```python
from build123d import *

# Parameters (mm, degrees)
SKETCH_W     = 13
SKETCH_H     = 10
PAD_DEPTH    = 12
POCKET_DEPTH = 8.5
SKETCH002_W  = 3
SKETCH002_H  = 10
PAD001_DEPTH = 10


with BuildPart() as part:
    # Sketch → Pad (new body)
    with BuildSketch(Plane.XZ):
        with Locations((0, -3)):
            Rectangle(SKETCH_W, SKETCH_H)
    extrude(amount=PAD_DEPTH)

    # Sketch001 → Pocket (cut)
    with BuildSketch(Plane(origin=(0, 0, 0), x_dir=(-1, 0, 0), z_dir=(0, 1, 0))):
        Polygon((-1.5, 5.906373), (1.5, 5.906373), (1.5, 0), (4.65, 0), (4.65, -8.83584), (-4.65, -8.83584), (-4.65, 0), (-1.5, 0), align=None)
    extrude(amount=-POCKET_DEPTH, mode=Mode.SUBTRACT)

    # Sketch002 (on Face7 of Pocket) → Pad001 (join)
    with BuildSketch(Plane(origin=(6.5, 0, 0), x_dir=(0, 0, 1), z_dir=(1, 0, 0))):
        with Locations((-6.5, 6)):
            Rectangle(SKETCH002_W, SKETCH002_H)
    pad001 = extrude(amount=PAD001_DEPTH)

    # Sketch003 (on DatumPlane) → Groove (revolve, cut)
    with BuildSketch(Plane.YZ.offset(11.5)):
        Polygon((-6, -5), (-8.636665, -5), (-7.5, -6.55), (-7.5, -10.559105), (-6, -10.559105), align=None)
    groove = revolve(axis=Axis((11.5, -6, -3.810725), (0, 0, -1)), mode=Mode.SUBTRACT)

    # Mirrored: Pad001, Groove across YZ
    add(pad001.mirror(Plane.YZ))
    add(groove.mirror(Plane.YZ), mode=Mode.SUBTRACT)


solid = part.part
```
Geometry check sheet. Reference: the model listing, model coordinates, mm. A direction names the side the tool comes from. Give positions to 0.01 mm unless a question says otherwise; leave off trailing zeros. Order: outer loops, then holes, each group sorted by start corner. A loop starts at its lowest first (then second) coordinate and runs counter-clockwise, first axis right, second up. Notation, with made-up numbers: (-29.5, 53) - (-11.5, 53) arc R22 cw to (-11.5, 89) - close; hole circle Ø3 at (-38.75, -13.75). An arc over 180 degrees is marked (long way). Write item = value, one per line. Start each with the question number.
1) Draft check along X on faces 1 (the flat face through (0, -12, -3)), 2 (the flat face through (-6.5, -6, -2)), 3 (the flat face through (-1.5, -4, 1)). Enter one of: released by +X, released by -X, zero draft, split by the parting line, or undercut.
2) Access from +Z, -Z, +X, -X, +Y, -Y to the whole of each face (thin tool, end or side, straight path). Record for faces 4 (the flat face through (14, -8, -5)), 5 (the flat face through (11, -1, -7)), 6 (the flat face through (3, -4, 0)), 7 (the flat face through (1.5, -4, 1)), 8 (the flat face through (-14, -8, -5)).
3) Section check D-D (z = -5.75). Enter the section's corners in (x, y).
4) Section check A-A (y = -6). Enter the section's corners in (x, z).
5) Gauge pin test, flat ends, axial feed: pin 1 Ø5 at (x, y) = (-12.5, -6) entering from +Z; pin 2 Ø2.5 at (x, z) = (9, -6) entering from -Y; pin 3 Ø4 at (y, z) = (-9, -4) entering from -X; pin 4 Ø1.6 at (y, z) = (-6, 1.5) entering from +X. Record the tip position at first contact, or that the pin passes through.
6) Section check B-B (x = -11.5). Enter the section's corners in (y, z).
7) Scan lines: L1, parallel to X at y = -6, z = -7.5; L2, parallel to Y at x = -11.5, z = -7.1; L3, parallel to X at y = -7.5, z = -1.75. Record each from-to range of solid material in increasing order.
8) Section check C-C (z = 0.5). Enter the section's corners in (x, y), then the cut area to 4 significant figures.
Geometry check:
q1.face_1 = zero draft
q1.face_2 = released by -X
q1.face_3 = undercut
q2.face_4 = +Z, +X, +Y, -Y
q2.face_5 = +Z, -Z, +X, +Y
q2.face_6 = -Z, +Y
q2.face_7 = +Z, -Z, +Y
q2.face_8 = +Z, -X, +Y, -Y
q3.outline = (-16.5, -11) - (-6.5, -11) - (-6.5, -12) - (6.5, -12) - (6.5, -11) - (16.5, -11) - (16.5, -1) - (6.5, -1) - (6.5, 0) - (4.65, 0) - (4.65, -8.5) - (-4.65, -8.5) - (-4.65, 0) - (-6.5, 0) - (-6.5, -1) - (-16.5, -1) - close; hole circle Ø4.17 at (-11.5, -6); hole circle Ø4.17 at (11.5, -6)
q4.outline = (-16.5, -8) - (-13, -8) - (-13, -6.55) - (-14.14, -5) - (-16.5, -5) - close; (-10, -8) - (-4.65, -8) - (-4.65, 0) - (-1.5, 0) - (-1.5, 2) - (-6.5, 2) - (-6.5, -5) - (-8.86, -5) - (-10, -6.55) - close; (1.5, 0) - (4.65, 0) - (4.65, -8) - (10, -8) - (10, -6.55) - (8.86, -5) - (6.5, -5) - (6.5, 2) - (1.5, 2) - close; (13, -8) - (16.5, -8) - (16.5, -5) - (14.14, -5) - (13, -6.55) - close
q5.pin_1 = -5
q5.pin_2 = -11
q5.pin_3 = -16.5
q5.pin_4 = 6.5
q6.outline = (-11, -8) - (-7.5, -8) - (-7.5, -6.55) - (-8.64, -5) - (-11, -5) - close; (-4.5, -8) - (-1, -8) - (-1, -5) - (-3.36, -5) - (-4.5, -6.55) - close
q7.L1 = -16.5 to -13, -10 to -4.65, 4.65 to 10, 13 to 16.5
q7.L2 = -11 to -7.5, -4.5 to -1
q7.L3 = -6.5 to -4.65, 4.65 to 6.5
q8.outline = (-6.5, -12) - (6.5, -12) - (6.5, 0) - (1.5, 0) - (1.5, -8.5) - (-1.5, -8.5) - (-1.5, 0) - (-6.5, 0) - close
q8.area = 130.5 mm2
